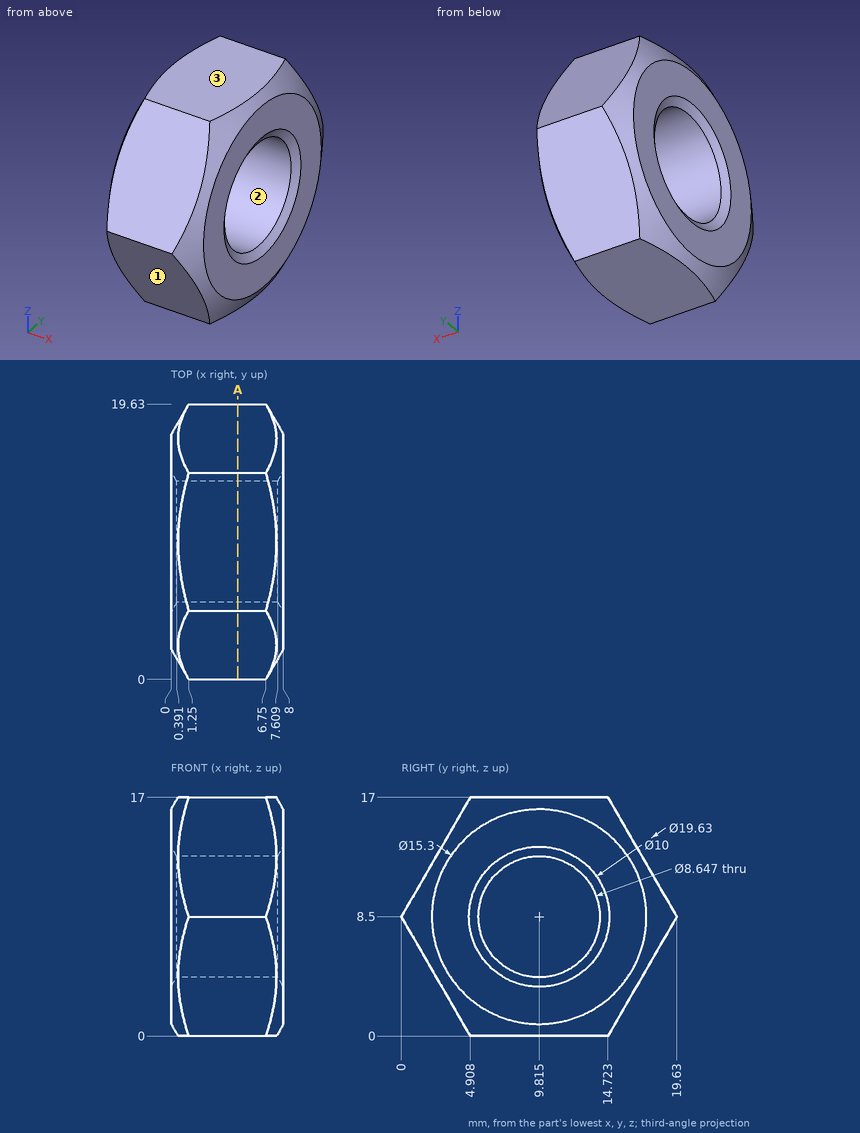
The drawing under review shows one solid part. Ordinate dimensions are in mm from its lowest x, y, z. Round coordinates to 2 decimals unless told otherwise and drop trailing zeros. Loops run counter-clockwise (first coordinate to the right, second up) from the corner with the lowest first, then second, coordinate; pieces in that order, holes last. Notation, with made-up numbers: (-2, 56) - (3, 56) arc R16 cw to (3, 68) - close; hole circle Ø10 at (30.5, -4). An arc over 180 degrees is marked (long way). Use a Markdown table: item, result. Add a question column.
Q1. Insertion check: pin 1 Ø4 at (x, y) = (2.5, 3.5) entering from -Z; pin 2 Ø1.5 at (x, z) = (6.5, 6.5) entering from +Y; pin 3 Ø4 at (x, z) = (2, 5) entering from -Y (1 decimal). Each pin has a flat end and moves straight along its axis. Give the tip position at first contact, or say it passes through.
Q2. For probe 1 along Y at (x, z) = (7.5, 6) (1 decimal); probe 2 along Z at (x, y) = (0.5, 11) (1 decimal); probe 3 along Z at (x, y) = (3, 7.25), list the stretches that pass through material, from the lowest coordinate up.
Q3. Add section A-A (x = 4.75). State the section outline as (y, z) points (1 decimal).
Q4. The part is to be moulded in two halves that separate along Y. For the marked faces 1, 2 and 3, say which applies: pulls with the +Y half, pulls with the -Y half, needs draft (parallel to the pull), parting line crosses it, or undercut.
Worked answers:
| question | item | result |
|---|---|---|
| 1 | pin 1 | z = 0 |
| 1 | pin 2 | y = 18.91 |
| 1 | pin 3 | y = 0.9 |
| 2 | probe 1 | 1.7 to 6.3, 13.3 to 18 |
| 2 | probe 2 | 0.1 to 4.3, 12.7 to 16.9 |
| 2 | probe 3 | 0 to 5.02, 11.98 to 17 |
| 3 | outline | (0, 8.5) - (4.9, 0) - (14.7, 0) - (19.6, 8.5) - (14.7, 17) - (4.9, 17) - close; hole circle Ø8.6 at (9.8, 8.5) |
| 4 | face 1 | pulls with the -Y half |
| 4 | face 2 | undercut |
| 4 | face 3 | needs draft |
